Verification items for this drawing (mm, ordinates from the low corner). A direction names the side the tool comes from. Give positions to 0.01 mm unless a question says otherwise; leave off trailing zeros. Write each loop counter-clockwise with the first axis right and the second up, starting at its lowest first coordinate (ties: lowest second). Pieces come first, ordered by that corner, then holes. Notation, with made-up numbers: (83, 2) -> (136, 2) arc R20 cw to (136, 15) -> close; hole circle Ø10 at (46.25, 51.25). An arc over 180 degrees is marked (long way). Answer as a JSON object with one key per item and string values.
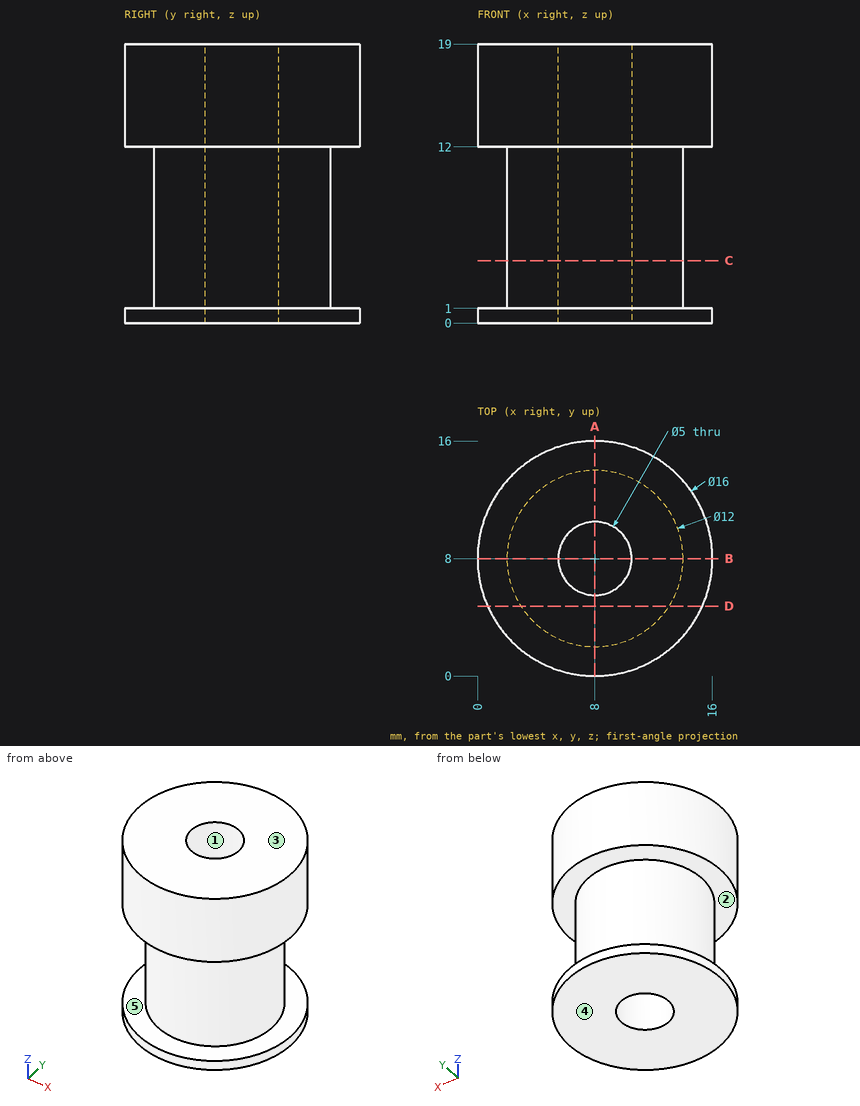
1. Scan lines: L1, parallel to Z at x = 13.25, y = 4.5; L2, parallel to Y at x = 8, z = 5; L3, parallel to X at y = 6.5, z = 10.5. Record each from-to range of solid material in increasing order. Write a range as [from, to].
Determined:
{"L1": "[0, 1], [12, 19]", "L2": "[2, 5.5], [10.5, 14]", "L3": "[2.19, 6], [10, 13.81]"}
2. Sectioned sample at A-A, the plane x = 8. Enter the section's corners in (y, z).
Determined:
{"outline": "(0, 0) -> (5.5, 0) -> (5.5, 19) -> (0, 19) -> (0, 12) -> (2, 12) -> (2, 1) -> (0, 1) -> close; (10.5, 0) -> (16, 0) -> (16, 1) -> (14, 1) -> (14, 12) -> (16, 12) -> (16, 19) -> (10.5, 19) -> close"}
3. Access from +Z, -Z, +X, -X, +Y, -Y to the whole of each face (thin tool, end or side, straight path). Record for the marked faces 1 and 2.
Determined:
{"face 1": "+Z, -Z", "face 2": "none"}
4. Mould release check, pull along Z, two halves, no side actions. Record for the marked faces 3, 4 and 5: released by +Z, released by -Z, zero draft, split by the parting line, or undercut.
Determined:
{"face 3": "released by +Z", "face 4": "released by -Z", "face 5": "undercut"}
5. Go/stop test with flat-tipped pins: P1, Ø1, axis at x = 5, z = 4.5, coming from the +Y side; P2, Ø3, axis at y = 3, z = 5.5, coming from the -X side; P3, Ø1.5, axis at x = 7.5, z = 3, coming from the +Y side. Record where each tip stops, or that it passes through.
Determined:
{"P1": "y = 13.45", "P2": "x = 3.13", "P3": "y = 14"}
6. Sectioned sample at D-D, the plane y = 4.75. Enter the section's corners in (x, z), plus the area to 3 significant figures.
Determined:
{"outline": "(0.69, 0) -> (15.31, 0) -> (15.31, 1) -> (13.04, 1) -> (13.04, 12) -> (15.31, 12) -> (15.31, 19) -> (0.69, 19) -> (0.69, 12) -> (2.96, 12) -> (2.96, 1) -> (0.69, 1) -> close", "area": "228 mm^2"}
7. Sectioned sample at C-C, the plane z = 4.25. Enter the section's corners in (x, y), plus the area to 3 significant figures.
Determined:
{"outline": "circle Ø12 at (8, 8); hole circle Ø5 at (8, 8)", "area": "93.5 mm^2"}
